Part print with two shaded views. Sizes in mm from the minimum x, y, z corner. A direction names the side the tool comes from. Give positions to 0.01 mm unless a question says otherwise; leave off trailing zeros. Order: outer loops, then holes, each group sorted by start corner. A loop starts at its lowest first (then second) coordinate and runs counter-clockwise, first axis right, second up. Notation, with made-up numbers: M 72,55 L 83,55 A10 ccw 83,67 Z; hole C 77.25,16 d5. An arc over 180 degrees is marked long. Answer as CSV lines item,"result".
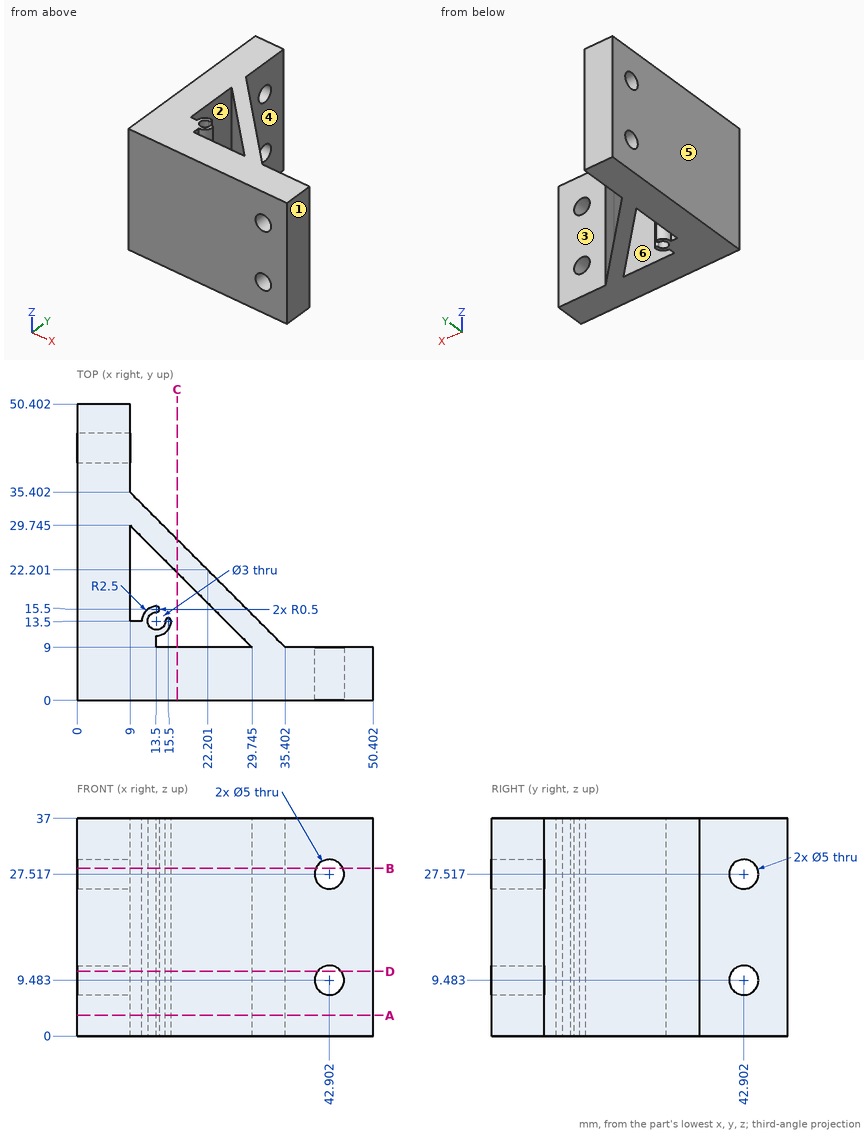
Item 1: Band-saw the part on C-C (x = 17). Give the cut face in (y, z) (3 decimals).
Geometry says:
outline,"M 0,0 L 9,0 L 9,37 L 0,37 Z; M 21.745,0 L 27.402,0 L 27.402,37 L 21.745,37 Z"
Item 2: Band-saw the part on D-D (z = 11). Give the cut face in (x, y) (3 decimals), and give its area (3 significant figures).
Geometry says:
outline,"M 0,0 L 40.915,0 L 40.915,9 L 35.402,9 L 9,35.402 L 9,40.915 L 0,40.915 Z; M 0,44.889 L 9,44.889 L 9,50.402 L 0,50.402 Z; M 44.889,0 L 50.402,0 L 50.402,9 L 44.889,9 Z; hole M 9,13.5 L 11,13.5 A2.5 cw 13.5,16 A0.5 cw 13.5,15 A1.5 ccw long 15,13.5 A0.5 cw 16,13.5 A2.5 cw 13.5,11 L 13.5,9 L 29.745,9 L 9,29.745 Z"
area,"914 mm2"
Item 3: Probe line 1 along X through (y, z) = (12.5, 7.5) (1 decimal); line 2 along X through (y, z) = (45, 17). List the from-to ranges inside material, lowest first. Write a range as from..to.
Geometry says:
line 1,"x = 0..12.4, 14.6..15.8, 26.2..31.9"
line 2,"x = 0..9"
Item 4: 3-axis set-ups, long thin cutter, end or side, ignore diameter. For the marked faces 1, 2 and 3: which of +Z, -Z, +X, -X, +Y, -Y reach the whole face in a straight line?
Geometry says:
face 1,"+Z, -Z, +X, +Y, -Y"
face 2,"+Z, -Z"
face 3,"+Z, -Z, +X, +Y"
Item 5: Pull direction X, two halves, no side cores. Call the marked faces 4, 5 and 6: released by +X, released by -X, zero draft, split by the parting line, or undercut.
Geometry says:
face 4,"released by +X"
face 5,"released by -X"
face 6,"undercut"
Item 6: Band-saw the part on B-B (z = 28.5). Give the cut face in (x, y) (1 decimal).
Geometry says:
outline,"M 0,0 L 40.6,0 L 40.6,9 L 35.4,9 L 9,35.4 L 9,40.6 L 0,40.6 Z; M 0,45.2 L 9,45.2 L 9,50.4 L 0,50.4 Z; M 45.2,0 L 50.4,0 L 50.4,9 L 45.2,9 Z; hole M 9,13.5 L 11,13.5 A2.5 cw 13.5,16 A0.5 cw 13.5,15 A1.5 ccw long 15,13.5 A0.5 cw 16,13.5 A2.5 cw 13.5,11 L 13.5,9 L 29.7,9 L 9,29.7 Z"
Item 7: Drop flat-ended pins along their axis: pin 1 (5 mm diameter, centred on x = 18.5, z = 18, fed in from +Y); pin 2 (12 mm diameter, centred on x = 23, z = 33, fed in from +Y); pin 3 (1.8 mm diameter, centred on x = 13.5, y = 13.5, fed in from +Z); pin 4 (10 mm diameter, centred on y = 29.5, z = 12, fed in from +X). Give the stop position or say it passes through.
Geometry says:
pin 1,"stops at y = 28.4"
pin 2,"stops at y = 27.4"
pin 3,"passes through"
pin 4,"stops at x = 19.9"
Item 8: Band-saw the part on A-A (z = 3.5). Give the cut face in (x, y) (3 decimals), and give its area (3 significant figures).
Geometry says:
outline,"M 0,0 L 50.402,0 L 50.402,9 L 35.402,9 L 9,35.402 L 9,50.402 L 0,50.402 Z; hole M 9,13.5 L 11,13.5 A2.5 cw 13.5,16 A0.5 cw 13.5,15 A1.5 ccw long 15,13.5 A0.5 cw 16,13.5 A2.5 cw 13.5,11 L 13.5,9 L 29.745,9 L 9,29.745 Z"
area,"985 mm2"
